Design review of the part built by this model. Coordinates are the model's own, in mm. Face numbers are marked on the shaded views. A direction names the side the tool comes from. Give positions to 0.01 mm unless a question says otherwise; leave off trailing zeros. Loops run counter-clockwise (first coordinate to the right, second up) from the corner with the lowest first, then second, coordinate; pieces in that order, holes last. Notation, with made-up numbers: (-32, -9) - (-10, -9) arc R17 cw to (-10, 13) - close; hole circle Ø11 at (66, -18.75). An arc over 180 degrees is marked (long way). Put each result on its own line as item: value. Start each with the question number.
```python
from build123d import *

# Parameters (mm, degrees)
SKETCH1_W           = 55
SKETCH1_H           = 35
BOSS_EXTRUDE1_DEPTH = 10
SKETCH2_W           = 22
SKETCH2_H           = 10
CUT_EXTRUDE1_DEPTH  = 34
CUT_EXTRUDE6_DEPTH  = 66.954529791
CUT_EXTRUDE7_DEPTH  = 66.954529791
SKETCH11_W          = 8
SKETCH11_H          = 22
BOSS_EXTRUDE3_DEPTH = 10
SKETCH12_R          = 1.45
CUT_EXTRUDE8_DEPTH  = 66.954529791
SKETCH13_R          = 1.95
CUT_EXTRUDE9_DEPTH  = 11
FILLET4_R           = 4
FILLET5_R           = 3
FILLET6_R           = 6
FILLET7_R           = 4
SKETCH14_W          = 8
SKETCH14_H          = 10
BOSS_EXTRUDE4_DEPTH = 2
SKETCH15_R          = 1.45
CUT_EXTRUDE10_DEPTH = 12
FILLET8_R           = 3


with BuildPart() as part:
    # Sketch1 → Boss-Extrude1 (new body)
    with BuildSketch(Plane(origin=(0, 0, 0), x_dir=(1, 0, 0), z_dir=(0, 1, 0))):
        with Locations((27.5, -17.5)):
            Rectangle(SKETCH1_W, SKETCH1_H)
    extrude(amount=BOSS_EXTRUDE1_DEPTH)

    # Sketch2 → Cut-Extrude1 (cut)
    with BuildSketch(Plane(origin=(55, 0, 0), x_dir=(0, 0, -1), z_dir=(1, 0, 0))):
        with Locations((-17.5, 5)):
            Rectangle(SKETCH2_W, SKETCH2_H)
    extrude(amount=-CUT_EXTRUDE1_DEPTH, mode=Mode.SUBTRACT)

    # Sketch9 → Cut-Extrude6 (cut, through all)
    with BuildSketch(Plane(origin=(0, 0, 0), x_dir=(-1, 0, 0), z_dir=(0, -1, 0))):
        Polygon((0, -12), (-18, 0), (0, 0), align=None)
        Polygon((0, -23), (-18, -35), (0, -35), align=None)
    extrude(amount=-CUT_EXTRUDE6_DEPTH, mode=Mode.SUBTRACT)

    # Sketch10 → Cut-Extrude7 (cut, through all)
    with BuildSketch(Plane(origin=(0, 0, 0), x_dir=(-1, 0, 0), z_dir=(0, -1, 0))):
        Polygon((-21, -6.5), (-7.444558288, -15), (-7.444558288, -20), (-21, -28.5), align=None)
    extrude(amount=-CUT_EXTRUDE7_DEPTH, mode=Mode.SUBTRACT)

    # Sketch11 → Boss-Extrude3 (add)
    with BuildSketch(Plane(origin=(0, 0, 0), x_dir=(-1, 0, 0), z_dir=(0, -1, 0))):
        with Locations((-33, -17.5)):
            Rectangle(SKETCH11_W, SKETCH11_H)
    extrude(amount=-BOSS_EXTRUDE3_DEPTH)

    # Sketch12 → Cut-Extrude8 (cut, through all)
    with BuildSketch(Plane.XY.offset(35)):
        with Locations((50, 5)):
            Circle(SKETCH12_R)
    extrude(amount=-CUT_EXTRUDE8_DEPTH, mode=Mode.SUBTRACT)

    # Sketch13 → Cut-Extrude9 (cut)
    with BuildSketch(Plane.ZY):
        with Locations((17.5, 5)):
            Circle(SKETCH13_R)
    extrude(amount=-CUT_EXTRUDE9_DEPTH, mode=Mode.SUBTRACT)

    # Fillet4
    fillet4_edges = [part.edges().sort_by_distance(p)[0] for p in [
        (55, 10, 31.75),
        (55, 0, 3.25),
        (55, 10, 3.25),
        (55, 0, 31.75),
    ]]
    fillet(fillet4_edges, radius=FILLET4_R)

    # Fillet5
    fillet5_edges = [part.edges().sort_by_distance(p)[0] for p in [
        (0, 5, 12),
        (0, 5, 23),
    ]]
    fillet(fillet5_edges, radius=FILLET5_R)

    # Fillet6
    fillet6_edges = [part.edges().sort_by_distance(p)[0] for p in [
        (18, 5, 0),
        (18, 5, 35),
    ]]
    fillet(fillet6_edges, radius=FILLET6_R)

    # Fillet7
    fillet7_edges = [part.edges().sort_by_distance(p)[0] for p in [
        (37, 5, 28.5),
        (37, 5, 6.5),
    ]]
    fillet(fillet7_edges, radius=FILLET7_R)

    # Sketch14 → Boss-Extrude4 (add)
    with BuildSketch(Plane.XY.offset(35)):
        with Locations((27, 5)):
            Rectangle(SKETCH14_W, SKETCH14_H)
    extrude(amount=BOSS_EXTRUDE4_DEPTH)

    # Sketch15 → Cut-Extrude10 (cut)
    with BuildSketch(Plane.XY.offset(37)):
        with Locations((27, 5)):
            Circle(SKETCH15_R)
    extrude(amount=-CUT_EXTRUDE10_DEPTH, mode=Mode.SUBTRACT)

    # Fillet8
    # the kernel refuses this fillet: 3 mm, written as the material it adds along each edge
    with BuildSketch(Plane(origin=(23, 0, 35), x_dir=(0, 0, 1), z_dir=(0, 1, 0))) as fillet8_piece_1:
        with BuildLine():
            CenterArc((3, -2.828427125), FILLET8_R, 109.471220634, 70.528779366)
            Line((0, -2.828427125), (-0.06, -2.828427125))
            Line((-0.06, -2.828427125), (-0.06, 0))
            Line((-0.06, 0), (0, 0.06))
            ThreePointArc((0, 0.06), (1, 0.06), (1.98, 0.056568542))
            Line((1.98, 0.056568542), (2, 0))
        make_face()
    extrude(amount=10)
    with BuildSketch(Plane(origin=(31, 10, 35), x_dir=(1, 0, 0), z_dir=(0, -1, 0))) as fillet8_piece_2:
        with BuildLine():
            CenterArc((2.828427125, 3), FILLET8_R, 199.471220634, 70.528779366)
            Line((0, 2), (-0.056568542, 1.98))
            ThreePointArc((-0.056568542, 1.98), (-0.06, 1), (-0.06, 0))
            Line((-0.06, 0), (0, -0.06))
            Line((0, -0.06), (2.828427125, -0.06))
            Line((2.828427125, -0.06), (2.828427125, 0))
        make_face()
    extrude(amount=10)


solid = part.part
```
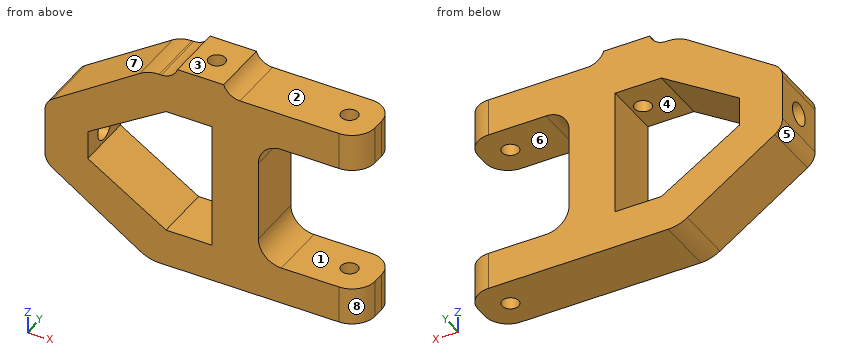
Item 1: For P1, Ø4, axis at x = 50, y = 5, coming from the +Z side; P2, Ø1.5, axis at x = 15, y = 6.5, coming from the -Z side; P3, Ø2.5, axis at x = 27, y = 5, coming from the +Z side; P4, Ø1.5, axis at x = 8, z = 29.5, coming from the +Y side, all flat-tipped, find the tip position at first contact; note any pin that passes through.
Item 2: Machinability: for the marked faces 1, 2, 3 and 4, which of the approach directions +Z, -Z, +X, -X, +Y, -Y give a long, thin tool a straight path to every point of the face, cutting with its end or side? Answer none if there is none.
Item 3: Consider section A-A (x = 50). State the section outline as (y, z) points, plus the area to 3 significant figures.
Item 4: Consider section C-C (x = 44). State the section outline as (y, z) points.
Item 5: For L1, parallel to X at y = 1.25, z = 15.5; L2, parallel to Y at x = 50, z = 2.25; L3, parallel to Z at x = 52.5, y = 5.75, list the stretches that pass through material, from the lowest coordinate up. Write a range as from..to.
Item 6: Consider section D-D (z = 4.5). State the section outline as (x, y) points, plus the area to 3 significant figures.
Item 7: Mouldability with a two-part tool opening along Z and no side actions: class the marked faces 5, 6, 7 and 8 as pulls with the +Z half, pulls with the -Z half, needs draft (parallel to the pull), parting line crosses it, or undercut.
Item 8: Consider section B-B (z = 17.5). State the section outline as (x, y) points, plus the area to 3 significant figures.
Geometry says:
1. P1: stops at z = 35
1. P2: stops at z = 1.5
1. P3: stops at z = 6.5
1. P4: passes through
2. face 1: +X, +Y, -Y
2. face 2: +Z, +X, +Y, -Y
2. face 3: +Z, +X, -X, +Y, -Y
2. face 4: +Y, -Y
3. outline: (0, 0) - (3.55, 0) - (3.55, 6.5) - (0, 6.5) - close; (0, 28.5) - (3.55, 28.5) - (3.55, 35) - (0, 35) - close; (6.45, 0) - (10, 0) - (10, 6.5) - (6.45, 6.5) - close; (6.45, 28.5) - (10, 28.5) - (10, 35) - (6.45, 35) - close
3. area: 92.3 mm2
4. outline: (0, 0) - (10, 0) - (10, 6.5) - (0, 6.5) - close; (0, 28.5) - (10, 28.5) - (10, 35) - (0, 35) - close
5. L1: x = 0..7.44, 29..37
5. L2: y = 0..3.55, 6.45..10
5. L3: z = 0..6.5, 28.5..35
6. outline: (11.25, 0) - (51, 0) arc R4 ccw to (55, 4) - (55, 6) arc R4 ccw to (51, 10) - (11.25, 10) - close; hole circle Ø2.9 at (50, 5)
6. area: 424 mm2
7. face 5: pulls with the -Z half
7. face 6: undercut
7. face 7: pulls with the +Z half
7. face 8: needs draft
8. outline: (0, 0) - (7.44, 0) - (7.44, 3.05) - (0, 3.05) - close; (0, 6.95) - (7.44, 6.95) - (7.44, 10) - (0, 10) - close; (29, 0) - (37, 0) - (37, 10) - (29, 10) - close
8. area: 125 mm2
